Model file for the job. Use its own axes, mm. A direction names the side the tool comes from. Round coordinates to 2 decimals unless told otherwise and drop trailing zeros. Loops run counter-clockwise (first coordinate to the right, second up) from the corner with the lowest first, then second, coordinate; pieces in that order, holes last. Notation, with made-up numbers: M -28.5,2.25 L 6.5,2.25 A17 ccw 6.5,13.25 Z; hole C 60.5,52 d8. An arc over 180 degrees is marked long. Use a Markdown table: item, result. Add a question column.
Q1. Cut at B-B (x = -1.25). Give the cut face in (y, z).
Q2. Tool access for faces 1 (the face through (0, 1, 1.27)), 2 (the face through (-0.317, 1.426, -1.252)): list every direction of +Z, -Z, +X, -X, +Y, -Y with a clear straight run to the whole face (end or side of a thin tool).
Q3. Pin check, flat tip, straight feed: pin 1 (2 mm diameter, centred on x = 0, z = -2, fed in from -Y). Stop position of the tip, or through.
Q4. Cut at D-D (y = 3). Give the cut face in (x, z), plus the area to 3 significant figures.
Q5. Probe line 1 (Z direction, x = 0.7, y = 1.5); line 2 (X direction, y = 1, z = -2.25); line 3 (X direction, y = 2.75, z = 0.5). List the from-to ranges inside material, lowest first. Write a range as from..to.
Q6. Cut at A-A (y = 0). Give the cut face in (x, z) (1 decimal), plus the area to 3 significant figures.
Q7. Cut at C-C (z = -1.7). Give the cut face in (x, y).
from build123d import *

# Parameters (mm, degrees)
F1_DEPTH = 1.27
F2_R     = 1.4605
F3_DEPTH = 2.54


with BuildPart() as f1:
    # F0 (on Top) → F1 (new body)
    with BuildSketch(Plane.XY):
        with BuildLine():
            Line((0, 4.572), (-1.731758, 0.79375))
            ThreePointArc((-1.731758, 0.79375), (0, -1.905), (1.731758, 0.79375))
            Line((1.731758, 0.79375), (0, 4.572))
        make_face()
    extrude(amount=F1_DEPTH)

    # F2 (on face) → F3 (join)
    with BuildSketch(Plane(origin=(0, 0, 0), x_dir=(1, 0, 0), z_dir=(0, 0, -1))):
        Circle(F2_R)
    extrude(amount=F3_DEPTH)


solid = f1.part
Checked values:
| question | item | result |
|---|---|---|
| 1 | outline | M -1.44,0 L -0.76,0 L -0.76,-2.54 L 0.76,-2.54 L 0.76,0 L 1.84,0 L 1.84,1.27 L -1.44,1.27 Z |
| 2 | face 1 | +Z, +X, -X, +Y, -Y |
| 2 | face 2 | -Z |
| 3 | pin 1 | stops at y = -1.46 |
| 4 | outline | M -0.72,0 L 0.72,0 L 0.72,1.27 L -0.72,1.27 Z |
| 4 | area | 1.83 mm^2 |
| 5 | line 1 | z = 0..1.27 |
| 5 | line 2 | x = -1.06..1.06 |
| 5 | line 3 | x = -0.84..0.84 |
| 6 | outline | M -1.9,0 L -1.5,0 L -1.5,-2.5 L 1.5,-2.5 L 1.5,0 L 1.9,0 L 1.9,1.3 L -1.9,1.3 Z |
| 6 | area | 12.3 mm^2 |
| 7 | outline | C 0,0 d2.92 |
